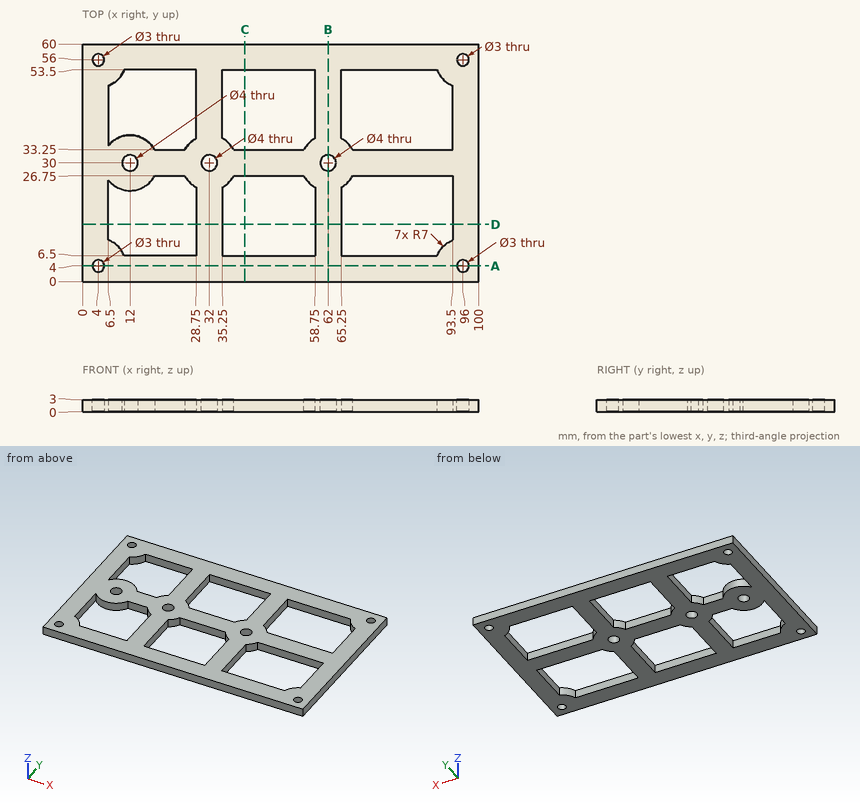
Here's the drawing with two shaded views (mm, measured from the low corner). I have some questions. Give positions to 0.01 mm unless a question says otherwise; leave off trailing zeros. Loops run counter-clockwise (first coordinate to the right, second up) from the corner with the lowest first, then second, coordinate; pieces in that order, holes last. Notation, with made-up numbers: M -16,89 L -5,89 A17 cw -5,114 Z; hole C 57,-19 d5. An arc over 180 degrees is marked long. Use one line per item in the form item = value. Start each with the question number.
Q1. If we section it at A-A (y = 4): Write out the boundary of the cut face in (x, z), then the cut area to 3 significant figures.
Q2. If we section it at D-D (y = 14.5): Write out the boundary of the cut face in (x, z), then the cut area to 3 significant figures.
Q3. I need wall thicknesses on line 1 along X through (y, z) = (18.5, 2.55); line 2 along Y through (x, z) = (4, 1.45); line 3 along Y through (x, z) = (68.5, 2.6). Which ranges of each line are inside material? Lowest first, please.
Q4. If we section it at B-B (x = 62): Write out the boundary of the cut face in (y, z), then the cut area to 3 significant figures.
Q5. If we section it at C-C (x = 41): Write out the boundary of the cut face in (y, z), then the cut area to 3 significant figures.
Taken from the geometry:
q1.outline = M 0,0 L 2.5,0 L 2.5,3 L 0,3 Z; M 5.5,0 L 94.5,0 L 94.5,3 L 5.5,3 Z; M 97.5,0 L 100,0 L 100,3 L 97.5,3 Z
q1.area = 282 mm^2
q2.outline = M 0,0 L 6.5,0 L 6.5,3 L 0,3 Z; M 28.75,0 L 35.25,0 L 35.25,3 L 28.75,3 Z; M 58.75,0 L 65.25,0 L 65.25,3 L 58.75,3 Z; M 93.5,0 L 100,0 L 100,3 L 93.5,3 Z
q2.area = 78.0 mm^2
q3.line_1 = 0 to 6.5, 28.75 to 35.25, 58.75 to 65.25, 93.5 to 100
q3.line_2 = 0 to 2.5, 5.5 to 54.5, 57.5 to 60
q3.line_3 = 0 to 6.5, 26.75 to 33.25, 53.5 to 60
q4.outline = M 0,0 L 28,0 L 28,3 L 0,3 Z; M 32,0 L 60,0 L 60,3 L 32,3 Z
q4.area = 168 mm^2
q5.outline = M 0,0 L 6.5,0 L 6.5,3 L 0,3 Z; M 26.75,0 L 33.25,0 L 33.25,3 L 26.75,3 Z; M 53.5,0 L 60,0 L 60,3 L 53.5,3 Z
q5.area = 58.5 mm^2
